Input: part model. Units: mm. Frame: model coordinates. Face numbers are marked on the shaded views. A direction names the side the tool comes from. Round coordinates to 2 decimals unless told otherwise and drop trailing zeros. Loops run counter-clockwise (first coordinate to the right, second up) from the corner with the lowest first, then second, coordinate; pieces in that order, holes last. Notation, with made-up numbers: (23, 36) - (69, 36) arc R19 cw to (69, 46) - close; hole circle Ø2 at (36, 19.25). An arc over 180 degrees is marked (long way). One line per question, with ' | ' between items. Start each with the question number.
from build123d import *

# Parameters (mm, degrees)
SKETCH1_R           = 10
BOSS_EXTRUDE2_DEPTH = 25
SKETCH2_R           = 10
SKETCH2_R_2         = 7
CUT_EXTRUDE1_DEPTH  = 9.8
SKETCH3_R           = 10
SKETCH3_R_2         = 6
CUT_EXTRUDE2_DEPTH  = 8
SKETCH4_R           = 4
CUT_EXTRUDE3_DEPTH  = 15
SKETCH5_R           = 2.75
CUT_EXTRUDE4_DEPTH  = 11
CUT_EXTRUDE5_DEPTH  = 8
SKETCH7_R           = 1.5
CUT_EXTRUDE6_DEPTH  = 4


with BuildPart() as part:
    # Sketch1 → Boss-Extrude2 (new body)
    with BuildSketch(Plane(origin=(0, 0, 0), x_dir=(1, 0, 0), z_dir=(0, 1, 0))):
        Circle(SKETCH1_R)
    extrude(amount=BOSS_EXTRUDE2_DEPTH)

    # Sketch2 → Cut-Extrude1 (cut)
    with BuildSketch(Plane(origin=(0, 25, 0), x_dir=(1, 0, 0), z_dir=(0, 1, 0))):
        Circle(SKETCH2_R)
        Circle(SKETCH2_R_2, mode=Mode.SUBTRACT)
    extrude(amount=-CUT_EXTRUDE1_DEPTH, mode=Mode.SUBTRACT)

    # Sketch3 → Cut-Extrude2 (cut)
    with BuildSketch(Plane.XZ):
        Circle(SKETCH3_R)
        Circle(SKETCH3_R_2, mode=Mode.SUBTRACT)
    extrude(amount=-CUT_EXTRUDE2_DEPTH, mode=Mode.SUBTRACT)

    # Sketch4 → Cut-Extrude3 (cut)
    with BuildSketch(Plane(origin=(0, 25, 0), x_dir=(1, 0, 0), z_dir=(0, 1, 0))):
        Circle(SKETCH4_R)
    extrude(amount=-CUT_EXTRUDE3_DEPTH, mode=Mode.SUBTRACT)

    # Sketch5 → Cut-Extrude4 (cut)
    with BuildSketch(Plane.XZ):
        Circle(SKETCH5_R)
    extrude(amount=-CUT_EXTRUDE4_DEPTH, mode=Mode.SUBTRACT)

    # Sketch6 → Cut-Extrude5 (cut)
    with BuildSketch(Plane.XZ):
        with BuildLine():
            Line((4.5, 0), (4.5, 3.968626967))
            ThreePointArc((4.5, 3.968626967), (6, 0), (4.5, -3.968626967))
            Line((4.5, -3.968626967), (4.5, 0))
        make_face()
    extrude(amount=-CUT_EXTRUDE5_DEPTH, mode=Mode.SUBTRACT)

    # Sketch7 → Cut-Extrude6 (cut)
    with BuildSketch(Plane(origin=(4.5, 0, 0), x_dir=(0, 0, -1), z_dir=(1, 0, 0))):
        with Locations((0, 4)):
            Circle(SKETCH7_R)
    extrude(amount=-CUT_EXTRUDE6_DEPTH, mode=Mode.SUBTRACT)


solid = part.part
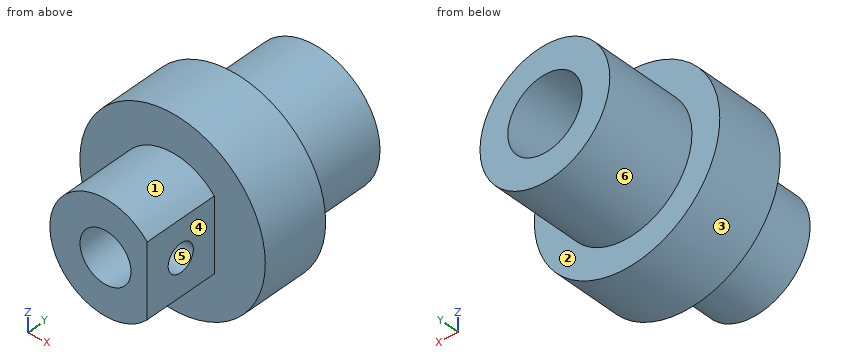
(1) Pin query (flat end, axial travel): P1, Ø1.8, axis at y = 4, z = 0, coming from the +X side; P2, Ø1, axis at y = 6.5, z = -4, coming from the -X side; P3, Ø2, axis at y = 10, z = -4, coming from the +X side. Return the tip coordinate at first contact, or that it passes through.
(2) Section B-B, the plane z = 0. Output: boundary loops of the cut face in (x, y), plus the area to 3 significant figures.
(3) Section D-D, the plane z = 5.5. Output: boundary loops of the cut face in (x, y).
(4) Pull-direction query (Z, two-part tool) for the marked faces 4, 5 and 6; classes: released by +Z, released by -Z, zero draft, split by the parting line, or undercut.
(5) Reachability of the marked faces 1, 2 and 3 from +Z, -Z, +X, -X, +Y, -Y: full face, straight path, thin tool, end or side. Return the list, or none.
(6) Line query: line 1 along Y through (x, z) = (3.05, 0); line 2 along X through (y, z) = (16.75, 0); line 3 along Z through (x, y) = (0, 6). Output: solid intervals per line, ascending. Write a range as from..to.
(7) Section C-C, the plane y = 14. Output: boundary loops of the cut face in (x, z).
(8) Section A-A, the plane x = 0. Output: boundary loops of the cut face in (y, z), plus the area to 3 significant figures.
Derived:
1) P1: stops at x = -2.6 | P2: stops at x = -4.87 | P3: stops at x = 9.54
2) outline: (-10, 8) - (-6, 8) - (-6, 0) - (-2.75, 0) - (-2.75, 10) - (-4, 10) - (-4, 25) - (-7, 25) - (-7, 15.2) - (-10, 15.2) - close; (2.75, 0) - (4.5, 0) - (4.5, 2.5) - (2.75, 2.5) - close; (2.75, 5.5) - (4.5, 5.5) - (4.5, 8) - (10, 8) - (10, 15.2) - (7, 15.2) - (7, 25) - (4, 25) - (4, 10) - (2.75, 10) - close | area: 185 mm²
3) outline: (-8.35, 8) - (-2.4, 8) - (-2.4, 0) - (2.4, 0) - (2.4, 8) - (8.35, 8) - (8.35, 15.2) - (4.33, 15.2) - (4.33, 25) - (-4.33, 25) - (-4.33, 15.2) - (-8.35, 15.2) - close
4) face 4: zero draft | face 5: undercut | face 6: split by the parting line
5) face 1: -Y | face 2: +Y | face 3: +Y, -Y
6) line 1: y = 0..2.5, 5.5..10 | line 2: x = -7..-4, 4..7 | line 3: z = -6..-2.75, 2.75..6
7) outline: circle Ø20 at (0, 0); hole circle Ø8 at (0, 0)
8) outline: (0, -6) - (8, -6) - (8, -10) - (15.2, -10) - (15.2, -7) - (25, -7) - (25, -4) - (10, -4) - (10, -2.75) - (0, -2.75) - close; (0, 2.75) - (10, 2.75) - (10, 4) - (25, 4) - (25, 7) - (15.2, 7) - (15.2, 10) - (8, 10) - (8, 6) - (0, 6) - close | area: 202 mm²
